Geometry check sheet. Reference: the model listing, model coordinates, mm. Face numbers are marked on the shaded views. Round coordinates to 2 decimals unless told otherwise and drop trailing zeros. Loops run counter-clockwise (first coordinate to the right, second up) from the corner with the lowest first, then second, coordinate; pieces in that order, holes last. Notation, with made-up numbers: (-13, 39.5) - (28, 39.5) arc R25 ccw to (28, 71.5) - close; hole circle Ø3 at (60, 43.5). An arc over 180 degrees is marked (long way). Answer as CSV lines item,"result". Start each with the question number.
1) Cross-section at C-C on z = 4. Record the boundary of the cut face in (x, y).
2) Cross-section at A-A on x = -21. Record the boundary of the cut face in (y, z).
3) Cross-section at B-B on z = 16.5. Record the boundary of the cut face in (x, y).
4) Depth check by flat-ended pin: P1, Ø12, axis at x = -29.5, z = 27.5, coming from the +Y side; P2, Ø1.5, axis at y = 18, z = 23.5, coming from the +X side; P3, Ø6, axis at x = -13.5, z = 11.5, coming from the +Y side. Enter the tip coordinate at first touch or a pass-through.
5) Cross-section at D-D on x = -7.5. Record the boundary of the cut face in (y, z).
6) Draft check along X on the marked faces 1, 2 and 3. Enter one of: released by +X, released by -X, zero draft, split by the parting line, or undercut.
7) Thickness scan on line 1 along X through (y, z) = (19, 17.5); line 2 along X through (y, z) = (-4, 17.5); line 3 along Y through (x, z) = (-23, 28). Record the ranges inside material, lowest first.
from build123d import *

# Parameters (mm, degrees)
F0_W     = 35.7145108283
F0_H     = 35.7145108283
F1_DEPTH = 10
F2_R     = 7.0075928512
F3_DEPTH = 25
F4_W     = 5.5791772902
F4_H     = 35.7145108283
F5_DEPTH = 25


with BuildPart() as f1:
    # F0 (on Front) → F1 (new body)
    with BuildSketch(Plane.XZ):
        with Locations((-17.8572554141, 17.8572554141)):
            Rectangle(F0_W, F0_H)
    extrude(amount=F1_DEPTH)

    # F2 (on face) → F3 (cut)
    with BuildSketch(Plane.XZ.offset(10)):
        with Locations((-17.8572554141, 17.8572554141)):
            Circle(F2_R)
    extrude(amount=-F3_DEPTH, mode=Mode.SUBTRACT)

    # F4 (on face) → F5 (join)
    with BuildSketch(Plane(origin=(0, 0, 0), x_dir=(-1, 0, 0), z_dir=(0, 1, 0))):
        with Locations((32.9249221832, 17.8572554141)):
            Rectangle(F4_W, F4_H)
    extrude(amount=F5_DEPTH)


solid = f1.part
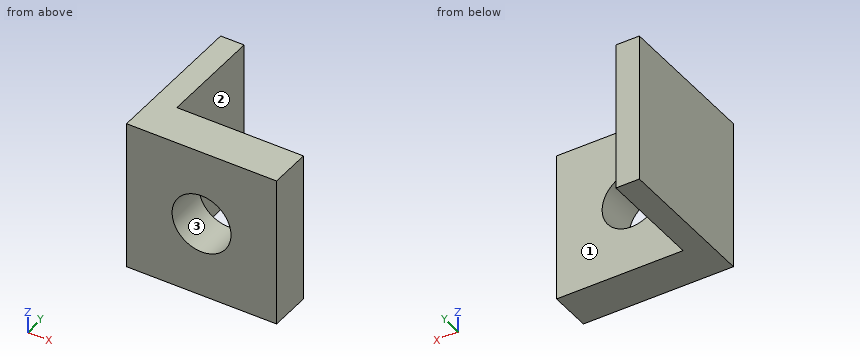
Answer block:
1,outline,"(-35.71, -10) - (0, -10) - (0, 0) - (-30.14, 0) - (-30.14, 25) - (-35.71, 25) - close"
2,outline,"(-10, 0) - (0, 0) - (0, 11.59) - (-10, 11.59) - close; (-10, 24.12) - (0, 24.12) - (0, 35.71) - (-10, 35.71) - close"
3,outline,"(-35.71, -10) - (-24.73, -10) - (-24.73, 0) - (-30.14, 0) - (-30.14, 25) - (-35.71, 25) - close; (-10.98, -10) - (0, -10) - (0, 0) - (-10.98, 0) - close"
4,P1,"stops at y = 25"
4,P2,"stops at x = -30.14"
4,P3,"stops at y = 0"
5,outline,"(-10, 0) - (0, 0) - (0, 35.71) - (-10, 35.71) - close"
6,face 1,"zero draft"
6,face 2,"released by +X"
6,face 3,"undercut"
7,line 1,"x = -35.71 to -30.14"
7,line 2,"x = -35.71 to -24.86, -10.86 to 0"
7,line 3,"y = -10 to 0"
